```python
from build123d import *

# Parameters (mm, degrees)
SKETCH1_W           = 130
SKETCH1_H           = 56
BOSS_EXTRUDE1_DEPTH = 3
SKETCH2_W           = 20
SKETCH2_H           = 36
CUT_EXTRUDE1_DEPTH  = 5
FILLET1_R           = 2


with BuildPart() as part:
    # Sketch1 → Boss-Extrude1 (new body)
    with BuildSketch(Plane.XY):
        Rectangle(SKETCH1_W, SKETCH1_H)
    extrude(amount=BOSS_EXTRUDE1_DEPTH)

    # Sketch2 → Cut-Extrude1 (cut)
    with BuildSketch(Plane.XY.offset(3)):
        with Locations((35, 0)):
            Rectangle(SKETCH2_W, SKETCH2_H)
        with Locations((-5, 0)):
            Rectangle(SKETCH2_W, SKETCH2_H)
        with Locations((-45, 0)):
            Rectangle(SKETCH2_W, SKETCH2_H)
    extrude(amount=-CUT_EXTRUDE1_DEPTH, mode=Mode.SUBTRACT)

    # Fillet1
    fillet1_edges = [part.edges().sort_by_distance(p)[0] for p in [
        (5, -18, 1.5),
        (-15, -18, 1.5),
        (-15, 18, 1.5),
        (5, 18, 1.5),
        (-55, 18, 1.5),
        (-35, 18, 1.5),
        (-35, -18, 1.5),
        (-55, -18, 1.5),
        (25, 18, 1.5),
        (45, 18, 1.5),
        (45, -18, 1.5),
        (25, -18, 1.5),
    ]]
    fillet(fillet1_edges, radius=FILLET1_R)


solid = part.part
```
The model under review builds one solid part; all positions refer to its coordinate system, in mm. A direction names the side the tool comes from. Coordinates: 2 decimals unless noted, no trailing zeros. Order: outer loops, then holes, each group sorted by start corner. A loop starts at its lowest first (then second) coordinate and runs counter-clockwise, first axis right, second up. Notation, with made-up numbers: (-14, 65) -> (31, 65) arc R20 ccw to (31, 99) -> close; hole circle Ø7 at (9, 11). An arc over 180 degrees is marked (long way). Answer in a Markdown table with one row per item. Add a question column.
Item 1: We need section B-B on z = 1.45. Write out the cut boundary in (x, y).
Item 2: Machinability: for faces 1 (the flat face through (35, -18, 2)), 2 (the flat face through (-1, -28, 1)), which of the approach directions +Z, -Z, +X, -X, +Y, -Y give a long, thin tool a straight path to every point of the face, cutting with its end or side? Answer none if there is none.
Item 3: To check wall thickness, follow probe 1 along X at (y, z) = (-9, 1.55); probe 2 along Y at (x, z) = (34, 2). State the ranges of each line that lie inside material, in increasing order.
Item 4: Mouldability with a two-part tool opening along X and no side actions: class faces 3 (the flat face through (65, 0, 1)), 4 (the flat face through (-55, 0, 2)), 5 (the flat face through (-65, 0, 1)) as +X half, -X half, draft (parallel to the pull), parting line (faces both ways), or undercut.
Item 5: We need section A-A on y = 6.5. Write out the cut boundary in (x, z).
Item 6: Clearance check with a flat-ended pin moving along its axis: pin 1 (10 mm diameter, centred on x = -41, y = 9, fed in from -Z). State where the tip first meets the part, or that it passes through.
Final values:
| question | item | result |
|---|---|---|
| 1 | outline | (-65, -28) -> (65, -28) -> (65, 28) -> (-65, 28) -> close; hole (-55, -16) arc R2 ccw to (-53, -18) -> (-37, -18) arc R2 ccw to (-35, -16) -> (-35, 16) arc R2 ccw to (-37, 18) -> (-53, 18) arc R2 ccw to (-55, 16) -> close; hole (-15, -16) arc R2 ccw to (-13, -18) -> (3, -18) arc R2 ccw to (5, -16) -> (5, 16) arc R2 ccw to (3, 18) -> (-13, 18) arc R2 ccw to (-15, 16) -> close; hole (25, -16) arc R2 ccw to (27, -18) -> (43, -18) arc R2 ccw to (45, -16) -> (45, 16) arc R2 ccw to (43, 18) -> (27, 18) arc R2 ccw to (25, 16) -> close |
| 2 | face 1 | +Z, -Z |
| 2 | face 2 | +Z, -Z, +X, -X, -Y |
| 3 | probe 1 | x = -65 to -55, -35 to -15, 5 to 25, 45 to 65 |
| 3 | probe 2 | y = -28 to -18, 18 to 28 |
| 4 | face 3 | +X half |
| 4 | face 4 | undercut |
| 4 | face 5 | -X half |
| 5 | outline | (-65, 0) -> (-55, 0) -> (-55, 3) -> (-65, 3) -> close; (-35, 0) -> (-15, 0) -> (-15, 3) -> (-35, 3) -> close; (5, 0) -> (25, 0) -> (25, 3) -> (5, 3) -> close; (45, 0) -> (65, 0) -> (65, 3) -> (45, 3) -> close |
| 6 | pin 1 | passes through |
